Input: part model. Units: mm. Frame: model coordinates. Face numbers are marked on the shaded views. A direction names the side the tool comes from. Coordinates: 2 decimals unless noted, no trailing zeros. Order: outer loops, then holes, each group sorted by start corner. A loop starts at its lowest first (then second) coordinate and runs counter-clockwise, first axis right, second up. Notation, with made-up numbers: (52, -39) -> (67, -39) arc R27 ccw to (67, -7) -> close; hole circle Ø1 at (-18, -18). An arc over 180 degrees is marked (long way). Write each question's results on one line, items separated by ' | '.
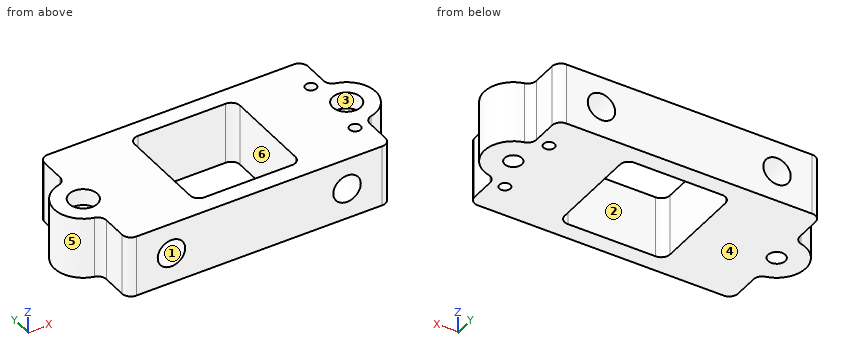
```python
from build123d import *

# Parameters (mm, degrees)
SKETCH1_W           = 93.6625
SKETCH1_H           = 40.64
SKETCH1_R           = 2.4892
SKETCH1_R_2         = 1.5875
BOSS_EXTRUDE1_DEPTH = 17.78
SKETCH6_R           = 3.96875
CUT_EXTRUDE4_DEPTH  = 104.635910312
CUT_EXTRUDE3_DEPTH  = 17.78
FILLET1_R           = 2.54
SKETCH3_R           = 4.064
CUT_EXTRUDE5_DEPTH  = 4.7752
CUT_EXTRUDE6_DEPTH  = 98.141100599


with BuildPart() as part:
    # Sketch1 → Boss-Extrude1 (new body)
    with BuildSketch(Plane.XY):
        with Locations((-46.83125, 0)):
            Rectangle(SKETCH1_W, SKETCH1_H)
        with Locations((-84.93125, 0)):
            Circle(SKETCH1_R, mode=Mode.SUBTRACT)
        with Locations((-8.73125, 0)):
            Circle(SKETCH1_R, mode=Mode.SUBTRACT)
        with Locations((-12.7, 10.16)):
            Circle(SKETCH1_R_2, mode=Mode.SUBTRACT)
        with Locations((-12.7, -10.16)):
            Circle(SKETCH1_R_2, mode=Mode.SUBTRACT)
    extrude(amount=-BOSS_EXTRUDE1_DEPTH)

    # Sketch6 → Cut-Extrude4 (cut, through all)
    with BuildSketch(Plane(origin=(0, 20.32, 0), x_dir=(1, 0, 0), z_dir=(0, 1, 0))):
        with Locations(Location((-72.23125, 8.89, 0), (0, 0, 270))):
            Circle(SKETCH6_R)
        with Locations(Location((-21.43125, 8.89, 0), (0, 0, 270))):
            Circle(SKETCH6_R)
    extrude(amount=-CUT_EXTRUDE4_DEPTH, mode=Mode.SUBTRACT)

    # Sketch5 → Cut-Extrude3 (cut)
    with BuildSketch(Plane.XY):
        with BuildLine():
            Line((-93.6625, -20.32), (-93.6625, 20.32))
            Line((-93.6625, 20.32), (-84.93125, 20.32))
            Line((-84.93125, 20.32), (-84.93125, 10.622546022))
            ThreePointArc((-84.93125, 10.622546022), (-85.477262526, 9.049137635), (-86.880552326, 8.152186482))
            ThreePointArc((-86.880552326, 8.152186482), (-93.31325, 0), (-86.880552326, -8.152186482))
            ThreePointArc((-86.880552326, -8.152186482), (-85.477262526, -9.049137635), (-84.93125, -10.622546022))
            Line((-84.93125, -10.622546022), (-84.93125, -20.32))
            Line((-84.93125, -20.32), (-93.6625, -20.32))
        make_face()
        with BuildLine():
            Line((0, -20.32), (0, 20.32))
            Line((0, 20.32), (-8.73125, 20.32))
            Line((-8.73125, 20.32), (-8.73125, 10.622546022))
            ThreePointArc((-8.73125, 10.622546022), (-8.185237474, 9.049137635), (-6.781947674, 8.152186482))
            ThreePointArc((-6.781947674, 8.152186482), (-0.34925, 0), (-6.781947674, -8.152186482))
            ThreePointArc((-6.781947674, -8.152186482), (-8.185237474, -9.049137635), (-8.73125, -10.622546022))
            Line((-8.73125, -10.622546022), (-8.73125, -20.32))
            Line((-8.73125, -20.32), (0, -20.32))
        make_face()
    extrude(amount=-CUT_EXTRUDE3_DEPTH, mode=Mode.SUBTRACT)

    # Fillet1
    fillet1_edges = [part.edges().sort_by_distance(p)[0] for p in [
        (-84.93125, 20.32, -8.89),
        (-84.93125, -20.32, -8.89),
        (-8.73125, 20.32, -8.89),
        (-8.73125, -20.32, -8.89),
    ]]
    fillet(fillet1_edges, radius=FILLET1_R)

    # Sketch3 → Cut-Extrude5 (cut)
    with BuildSketch(Plane.XY):
        with Locations((-84.93125, 0)):
            Circle(SKETCH3_R)
        with Locations((-8.73125, 0)):
            Circle(SKETCH3_R)
    extrude(amount=-CUT_EXTRUDE5_DEPTH, mode=Mode.SUBTRACT)

    # Sketch7 → Cut-Extrude6 (cut, through all)
    with BuildSketch(Plane.XY):
        with BuildLine():
            Line((-59.53125, -15.24), (-34.13125, -15.24))
            ThreePointArc((-34.13125, -15.24), (-32.335198776, -14.496051224), (-31.59125, -12.7))
            Line((-31.59125, -12.7), (-31.59125, 12.7))
            ThreePointArc((-31.59125, 12.7), (-32.335198776, 14.496051224), (-34.13125, 15.24))
            Line((-34.13125, 15.24), (-59.53125, 15.24))
            ThreePointArc((-59.53125, 15.24), (-61.327301224, 14.496051224), (-62.07125, 12.7))
            Line((-62.07125, 12.7), (-62.07125, -12.7))
            ThreePointArc((-62.07125, -12.7), (-61.327301224, -14.496051224), (-59.53125, -15.24))
        make_face()
    extrude(amount=-CUT_EXTRUDE6_DEPTH, mode=Mode.SUBTRACT)


solid = part.part
```
(1) Line query: line 1 along Y through (x, z) = (-12.7, -6.5); line 2 along X through (y, z) = (-12, -16); line 3 along Y through (x, z) = (-36, -10.5). Output: solid intervals per line, ascending. Write a range as from..to.
Return value:
line 1: -20.32..-11.75, -8.57..8.57, 11.75..20.32 | line 2: -84.93..-62.07, -31.59..-8.73 | line 3: -20.32..-15.24, 15.24..20.32
(2) Cut plane A-A, the plane x = -37. Return loops of the section in (y, z).
Return value:
outline: (-20.32, -17.78) -> (-15.24, -17.78) -> (-15.24, 0) -> (-20.32, 0) -> close; (15.24, -17.78) -> (20.32, -17.78) -> (20.32, 0) -> (15.24, 0) -> close
(3) Cut plane C-C, the plane y = -6.5. Return loops of the section in (x, z).
Return value:
outline: (-90.22, -17.78) -> (-62.07, -17.78) -> (-62.07, 0) -> (-90.22, 0) -> close; (-31.59, -17.78) -> (-3.44, -17.78) -> (-3.44, 0) -> (-31.59, 0) -> close; hole circle Ø7.94 at (-72.23, -8.89); hole circle Ø7.94 at (-21.43, -8.89)
(4) Cut plane D-D, the plane z = -8.89. Count the separate pieces of the cut face and the enclosed holes in it, plus the area to 3 significant figures.
Return value:
separate pieces: 3 | enclosed holes: 5 | area: 1,690 mm2
(5) Pin query (flat end, axial travel): P1, Ø5.5, axis at y = -14, z = -11.5, coming from the +X side; P2, Ø5.5, axis at x = -8.73, y = 0, coming from the +Z side; P3, Ø2, axis at y = -15.5, z = -14.5, coming from the -X side. Return the tip coordinate at first contact, or that it passes through.
Return value:
P1: x = -8.73 | P2: z = -4.78 | P3: x = -84.93
(6) Reachability of the marked faces 1, 2 and 3 from +Z, -Z, +X, -X, +Y, -Y: full face, straight path, thin tool, end or side. Return the list, or none.
Return value:
face 1: +Y, -Y | face 2: +Z, -Z | face 3: +Z
(7) Cut plane B-B, the plane z = -1.5. Return loops of the section in (x, y) (1 decimal).
Return value:
outline: (-86.9, -8.2) arc R2.5 cw to (-84.9, -10.6) -> (-84.9, -17.8) arc R2.5 ccw to (-82.4, -20.3) -> (-11.3, -20.3) arc R2.5 ccw to (-8.7, -17.8) -> (-8.7, -10.6) arc R2.5 cw to (-6.8, -8.2) arc R8.4 ccw to (-6.8, 8.2) arc R2.5 cw to (-8.7, 10.6) -> (-8.7, 17.8) arc R2.5 ccw to (-11.3, 20.3) -> (-82.4, 20.3) arc R2.5 ccw to (-84.9, 17.8) -> (-84.9, 10.6) arc R2.5 cw to (-86.9, 8.2) arc R8.4 ccw to start; hole circle Ø8.1 at (-84.9, 0); hole (-62.1, -12.7) arc R2.5 ccw to (-59.5, -15.2) -> (-34.1, -15.2) arc R2.5 ccw to (-31.6, -12.7) -> (-31.6, 12.7) arc R2.5 ccw to (-34.1, 15.2) -> (-59.5, 15.2) arc R2.5 ccw to (-62.1, 12.7) -> close; hole circle Ø3.2 at (-12.7, -10.2); hole circle Ø3.2 at (-12.7, 10.2); hole circle Ø8.1 at (-8.7, 0)
(8) Mould query, pull axis X, two halves, no side actions, for the marked faces 4, 5 and 6. Classes: +X half, -X half, draft (parallel to the pull), parting line (faces both ways), or undercut.
Return value:
face 4: draft | face 5: -X half | face 6: undercut
